from build123d import *

# Parameters (mm, degrees)
F0_R          = 2.2225
F1_DEPTH      = 40.64
F1_DEPTH_BACK = 40.64
F2_R          = 4.445
F2_R_2        = 2.2225
F3_DEPTH      = 3.81
F6_W          = 1.016
F6_H          = 12.7
F7_DEPTH      = 25.4
F7_DEPTH_BACK = 25.4


with BuildPart() as f1:
    # F0 (on Top) → F1 (new body, two sides)
    with BuildSketch(Plane.XY) as f1_sk:
        Circle(F0_R)
    extrude(amount=F1_DEPTH)
    extrude(f1_sk.sketch, amount=-F1_DEPTH_BACK)

    # F2 (on face) → F3 (join)
    with BuildSketch(Plane(origin=(0, 0, -40.64), x_dir=(1, 0, 0), z_dir=(0, 0, -1))):
        Circle(F2_R)
        Circle(F2_R_2, mode=Mode.SUBTRACT)
    extrude(amount=-F3_DEPTH)

    # F4 (on Front) → F5 (revolve, cut)
    with BuildSketch(Plane.XZ):
        with BuildLine():
            ThreePointArc((-1.778, 36.83), (-2.0915595064, 38.735), (-1.778, 40.64))
            Line((-1.778, 40.64), (-5.5500328927, 40.64))
            Line((-5.5500328927, 40.64), (-5.5500328927, 36.83))
            Line((-5.5500328927, 36.83), (-1.778, 36.83))
        make_face()
    revolve(axis=Axis((0, 0, 38.735), (0, 0, -1)), mode=Mode.SUBTRACT)

    # F6 (on Front) → F7 (cut, two sides)
    with BuildSketch(Plane.XZ) as f7_sk:
        with Locations((0, 34.6862748265)):
            Rectangle(F6_W, F6_H)
    extrude(amount=-F7_DEPTH, mode=Mode.SUBTRACT)
    extrude(f7_sk.sketch, amount=F7_DEPTH_BACK, mode=Mode.SUBTRACT)


solid = f1.part
Verification items for the finished model (mm, model axes). A direction names the side the tool comes from. Coordinates: 2 decimals unless noted, no trailing zeros. Order: outer loops, then holes, each group sorted by start corner. A loop starts at its lowest first (then second) coordinate and runs counter-clockwise, first axis right, second up. Notation, with made-up numbers: M 87.5,-3.75 L 107.5,-3.75 A28 ccw 107.5,25.25 Z; hole C -27,-15 d1. An arc over 180 degrees is marked long. Write each question's results on one line, items separated by ' | '.
1) Access from +Z, -Z, +X, -X, +Y, -Y to the whole of each face (thin tool, end or side, straight path). Record for faces 4 (the face through (-0.508, 0, 34)), 5 (the face through (-1, 0, 40.64)), 6 (the face through (2.12, 0.67, 0.52)).
Solved:
face 4: +Z, +Y, -Y | face 5: +Z, +X, -X, +Y, -Y | face 6: +Z
2) Section check C-C on x = 3.75. Record the cut outline in (y, z), plus the area to 3 significant figures.
Solved:
outline: M -2.39,-40.64 L 2.39,-40.64 L 2.39,-36.83 L -2.39,-36.83 Z | area: 18.2 mm²
3) Section check D-D on y = 3. Record the cut outline in (x, z), plus the area to 3 significant figures.
Solved:
outline: M -3.28,-40.64 L 3.28,-40.64 L 3.28,-36.83 L -3.28,-36.83 Z | area: 25.0 mm²
4) Scan lines: line 1 along Y through (x, z) = (0.5, 17.5); line 2 along Z through (x, y) = (-1.5, 3); line 3 along X through (y, z) = (0, 26.5). Record each from-to range of solid material in increasing order. Write a range as [from, to].
Solved:
line 1: y = [-2.17, 2.17] | line 2: z = [-40.64, -36.83] | line 3: x = [-2.22, 2.22]
5) Release check for a two-part mould opening along Z. For faces 1 (the face through (-2, 0, 36.83)), 2 (the face through (0.508, 0, 34)), 3 (the face through (2, 2, -36.83)) record: pulls with the +Z half, pulls with the -Z half, needs draft (parallel to the pull), parting line crosses it, or undercut.
Solved:
face 1: undercut | face 2: needs draft | face 3: pulls with the +Z half
6) Gauge pin test, flat ends, axial feed: pin 1 Ø0.5 at (x, y) = (-1.5, -1) entering from +Z; pin 2 Ø2 at (y, z) = (0.5, 32.5) entering from +X; pin 3 Ø3.5 at (y, z) = (-1, 32.5) entering from -X; pin 4 Ø1 at (y, z) = (2.5, 12.5) entering from -X. Record the tip position at first contact, or that the pin passes through.
Solved:
pin 1: stops at z = 40.64 | pin 2: stops at x = 2.22 | pin 3: stops at x = -2.22 | pin 4: stops at x = -0.97
7) Section check B-B on z = 16. Record the cut outline in (x, y) (1 decimal), plus the area to 3 significant figures.
Solved:
outline: C 0,0 d4.4 | area: 15.5 mm²
